from build123d import *

# Parameters (mm, degrees)
F0_W     = 2.413
F0_H     = 2.54
F0_R     = 4.7018325436
F1_DEPTH = 3.175
F2_DEPTH = 9.398
F3_DEPTH = 3.175


with BuildPart() as f1:
    # F0 (on Front) → F1 (new body, symmetric)
    with BuildSketch(Plane.XZ):
        Polygon((3.96875, -30.1625), (3.96875, 30.1625), (-3.96875, 30.1625), (-3.96875, 15.875), (-3.96875, 13.4112), (-3.96875, -30.1625), align=None)
        with Locations((0, 14.4846439362)):
            Rectangle(F0_W, F0_H, mode=Mode.SUBTRACT)
        with BuildLine():
            Line((-3.96875, 30.1625), (3.96875, 30.1625))
            ThreePointArc((3.96875, 30.1625), (0, 34.13125), (-3.96875, 30.1625))
        make_face()
        with BuildLine():
            ThreePointArc((-3.96875, -30.1625), (0, -34.13125), (3.96875, -30.1625))
            Line((3.96875, -30.1625), (-3.96875, -30.1625))
        make_face()
        with BuildLine():
            Line((-13.49375, 15.875), (-13.4827836254, 15.875))
            ThreePointArc((-13.4827836254, 15.875), (-26.0674995034, 14.699090169), (-13.49375, 13.4112))
            Line((-13.49375, 13.4112), (-13.49375, 15.875))
        make_face()
        with Locations((-19.7175624037, 14.6708265968)):
            Circle(F0_R, mode=Mode.SUBTRACT)
        with BuildLine():
            ThreePointArc((-13.3675624037, 14.6708265968), (-13.3964333415, 15.2756632514), (-13.4827836254, 15.875))
            Line((-13.4827836254, 15.875), (-13.49375, 15.875))
            Line((-13.49375, 15.875), (-13.49375, 13.4112))
            ThreePointArc((-13.49375, 13.4112), (-13.3991880573, 14.0378608645), (-13.3675624037, 14.6708265968))
        make_face()
        with BuildLine():
            Line((-3.96875, 13.4112), (-3.96875, 15.875))
            Line((-3.96875, 15.875), (-13.4827836254, 15.875))
            ThreePointArc((-13.4827836254, 15.875), (-13.3964333415, 15.2756632514), (-13.3675624037, 14.6708265968))
            ThreePointArc((-13.3675624037, 14.6708265968), (-13.3991880573, 14.0378608645), (-13.49375, 13.4112))
            Line((-13.49375, 13.4112), (-3.96875, 13.4112))
        make_face()
    extrude(amount=F1_DEPTH, both=True)

    # F0 (on Front) → F2 (join)
    with BuildSketch(Plane.XZ):
        with Locations((0, 14.4846439362)):
            Rectangle(F0_W, F0_H)
    extrude(amount=F2_DEPTH)

    # F0 (on Front) → F3 (join)
    with BuildSketch(Plane.XZ):
        with Locations((0, 14.4846439362)):
            Rectangle(F0_W, F0_H)
    extrude(amount=-F3_DEPTH)


solid = f1.part
Read the model definition and answer for the solid it produces. Units are mm, in the model's axes. A direction names the side the tool comes from. Round coordinates to 2 decimals unless told otherwise and drop trailing zeros. Order: outer loops, then holes, each group sorted by start corner. A loop starts at its lowest first (then second) coordinate and runs counter-clockwise, first axis right, second up.
1) The part is cut by section D-D on z = 20. Write down the section's boundary in (x, y) (3 decimals), plus the area to 3 significant figures.
2) The part is cut by section A-A on x = -16.5. Write down the section's boundary in (y, z) (3 decimals).
3) The part is cut by section C-C on x = 0. Write down the section's boundary in (y, z) (3 decimals), plus the area to 3 significant figures.
4) Straight lines are drawn through the part: L1, parallel to X at y = 0.5, z = 18.5; L2, parallel to X at y = -1, z = 7; L3, parallel to X at y = 2.75, z = 12. For each, find the intervals that lie inside material, in ascending order.
5) The mould has two halves that part along X. Classify faces 1 (the face through (-0.09, -0.04, -34.13)), 2 (the face through (-9, 0, 13.411)), 3 (the face through (-2, -3.175, 3)): released by +X, released by -X, zero draft, split by the parting line, or undercut.
6) For faces 4 (the face through (0, -6, 13.215)), 5 (the face through (1.206, -6, 14)), 6 (the face through (0, -6, 15.755)), 7 (the face through (-3.969, 0, 23)), determine the directions among +Z, -Z, +X, -X, +Y, -Y from which every point of the face is accessible in a straight line to the end or side of a thin tool.
7) Flat-ended cylindrical pins translate along their axes: pin 1 (15 mm diameter, centred on x = -8.5, z = -9, fed in from -Y) (3 decimals); pin 2 (3 mm diameter, centred on x = -8, y = -0.5, fed in from +Z) (3 decimals); pin 3 (1.9 mm diameter, centred on x = 0, y = -5, fed in from -Z). Find the tip coordinate at first contact, or state that the pin passes through.
Resolved:
1. outline: (-23.17, -3.175) - (-16.265, -3.175) - (-16.265, 3.175) - (-23.17, 3.175) - close; (-3.969, -3.175) - (3.969, -3.175) - (3.969, 3.175) - (-3.969, 3.175) - close
1. area: 94.3 mm2
2. outline: (-3.175, 9.196) - (3.175, 9.196) - (3.175, 11.242) - (-3.175, 11.242) - close; (-3.175, 18.099) - (3.175, 18.099) - (3.175, 20.145) - (-3.175, 20.145) - close
3. outline: (-9.398, 13.215) - (-3.175, 13.215) - (-3.175, -34.131) - (3.175, -34.131) - (3.175, 34.131) - (-3.175, 34.131) - (-3.175, 15.755) - (-9.398, 15.755) - close
3. area: 449 mm2
4. L1: x = -24.78 to -22.45, -16.99 to -14.65, -3.97 to 3.97
4. L2: x = -3.97 to 3.97
4. L3: x = -25.48 to -23.59, -15.85 to -13.96, -3.97 to 3.97
5. face 1: split by the parting line
5. face 2: undercut
5. face 3: zero draft
6. face 4: -Z, +X, -X, -Y
6. face 5: +Z, -Z, +X, -Y
6. face 6: +Z, +X, -X, -Y
6. face 7: +Z, +Y, -Y
7. pin 1: stops at y = -3.175
7. pin 2: stops at z = 15.875
7. pin 3: stops at z = 13.21
